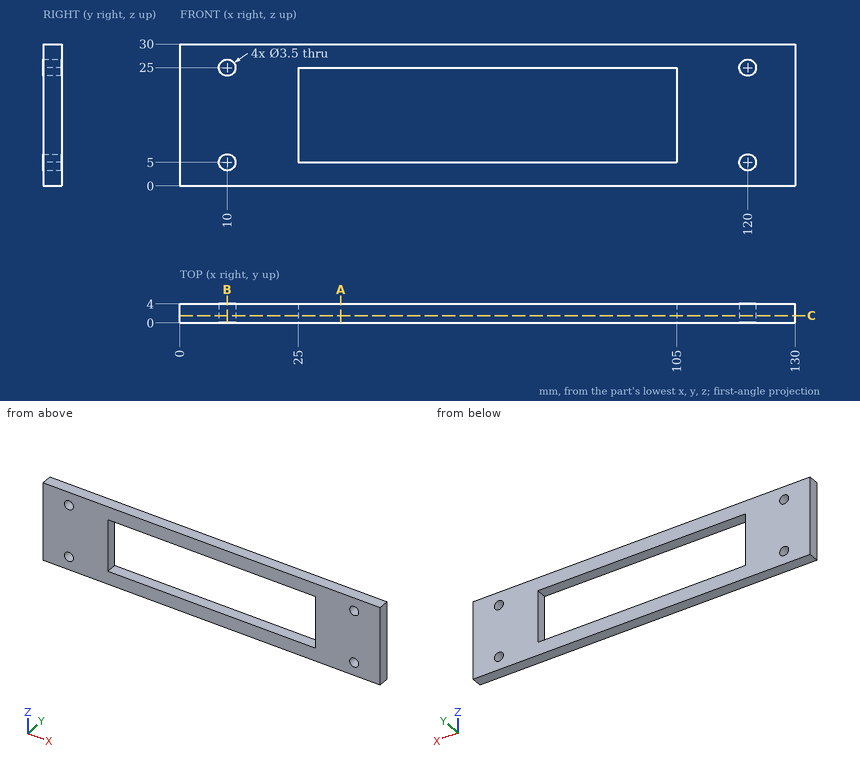
The figure shows three views and two pictorial views of one solid part (mm, origin at its lowest corner). Answer the questions. Coordinates: 2 decimals unless noted, no trailing zeros. Loops run counter-clockwise (first coordinate to the right, second up) from the corner with the lowest first, then second, coordinate; pieces in that order, holes last. Notation, with made-up numbers: (35.25, -12.75) -> (50.25, -12.75) arc R26 ccw to (50.25, 8.25) -> close; hole circle Ø2 at (26, -1). An arc over 180 degrees is marked (long way). Return JSON: item names as keys, results as strings. Group by question number.
(1) Find the intervals of material crossed by probe 1 along X at (y, z) = (1.05, 16); probe 2 along Z at (x, y) = (73, 1.4); probe 3 along X at (y, z) = (0.4, 4), in increasing order. Write a range as from..to.
(2) A cutting plane is placed at A-A on x = 34. Write down the section's boundary in (y, z).
(3) Given pin 1 Ø3 at (x, z) = (10, 5) entering from -Y, flat-ended and moving along its own axis, determine where the tip first touches the part or whether it passes through.
(4) A cutting plane is placed at C-C on y = 1.55. Write down the section's boundary in (x, z), and give its area (3 significant figures).
(5) A cutting plane is placed at B-B on x = 10. Write down the section's boundary in (y, z).
The answers:
{
 "1": {"probe 1": "x = 0..25, 105..130", "probe 2": "z = 0..5, 25..30", "probe 3": "x = 0..8.56, 11.44..118.56, 121.44..130"},
 "2": {"outline": "(0, 0) -> (4, 0) -> (4, 5) -> (0, 5) -> close; (0, 25) -> (4, 25) -> (4, 30) -> (0, 30) -> close"},
 "3": {"pin 1": "passes through"},
 "4": {"outline": "(0, 0) -> (130, 0) -> (130, 30) -> (0, 30) -> close; hole circle Ø3.5 at (10, 5); hole circle Ø3.5 at (10, 25); hole (25, 5) -> (105, 5) -> (105, 25) -> (25, 25) -> close; hole circle Ø3.5 at (120, 5); hole circle Ø3.5 at (120, 25)", "area": "2,260 mm^2"},
 "5": {"outline": "(0, 0) -> (4, 0) -> (4, 3.25) -> (0, 3.25) -> close; (0, 6.75) -> (4, 6.75) -> (4, 23.25) -> (0, 23.25) -> close; (0, 26.75) -> (4, 26.75) -> (4, 30) -> (0, 30) -> close"}
}
